Read the model definition and answer for the solid it produces. Units are mm, in the model's axes. A direction names the side the tool comes from. Round coordinates to 2 decimals unless told otherwise and drop trailing zeros. Loops run counter-clockwise (first coordinate to the right, second up) from the corner with the lowest first, then second, coordinate; pieces in that order, holes last. Notation, with made-up numbers: (-22, -4.75) - (-6, -4.75) arc R18 cw to (-6, 20.25) - close; hole circle Ø2 at (-22.75, 58). An arc over 180 degrees is marked (long way). Use one line per item in the form item = value. Start each with the question number.
```python
from build123d import *

# Parameters (mm, degrees)
SKETCH1_R           = 2.5
BOSS_EXTRUDE1_DEPTH = 300
SKETCH2_W           = 20
SKETCH2_H           = 180
CUT_EXTRUDE1_DEPTH  = 30


with BuildPart() as part:
    # Sketch1 → Boss-Extrude1 (new body)
    with BuildSketch(Plane(origin=(0, 0, 0), x_dir=(-1, 0, 0), z_dir=(0, 0, -1))):
        with BuildLine():
            Line((-20, 19), (-20, 13.2))
            Line((-20, 13.2), (-18.2, 13.2))
            Line((-18.2, 13.2), (-18.2, 14.95))
            ThreePointArc((-18.2, 14.95), (-18.053553391, 15.303553391), (-17.7, 15.45))
            Line((-17.7, 15.45), (-16.607106781, 15.45))
            ThreePointArc((-16.607106781, 15.45), (-16.415765065, 15.411939766), (-16.253553391, 15.303553391))
            Line((-16.253553391, 15.303553391), (-14.046446609, 13.096446609))
            ThreePointArc((-14.046446609, 13.096446609), (-13.938060234, 12.934234935), (-13.9, 12.742893219))
            Line((-13.9, 12.742893219), (-13.9, 7.257106781))
            ThreePointArc((-13.9, 7.257106781), (-13.938060234, 7.065765065), (-14.046446609, 6.903553391))
            Line((-14.046446609, 6.903553391), (-16.253553391, 4.696446609))
            ThreePointArc((-16.253553391, 4.696446609), (-16.415765065, 4.588060234), (-16.607106781, 4.55))
            Line((-16.607106781, 4.55), (-17.7, 4.55))
            ThreePointArc((-17.7, 4.55), (-18.053553391, 4.696446609), (-18.2, 5.05))
            Line((-18.2, 5.05), (-18.2, 6.8))
            Line((-18.2, 6.8), (-20, 6.8))
            Line((-20, 6.8), (-20, 1))
            ThreePointArc((-20, 1), (-19.707106781, 0.292893219), (-19, 0))
            Line((-19, 0), (-13.2, 0))
            Line((-13.2, 0), (-13.2, 1.8))
            Line((-13.2, 1.8), (-14.95, 1.8))
            ThreePointArc((-14.95, 1.8), (-15.303553391, 1.946446609), (-15.45, 2.3))
            Line((-15.45, 2.3), (-15.45, 3.392893219))
            ThreePointArc((-15.45, 3.392893219), (-15.411939766, 3.584234935), (-15.303553391, 3.746446609))
            Line((-15.303553391, 3.746446609), (-13.096446609, 5.953553391))
            ThreePointArc((-13.096446609, 5.953553391), (-12.934234935, 6.061939766), (-12.742893219, 6.1))
            Line((-12.742893219, 6.1), (-7.257106781, 6.1))
            ThreePointArc((-7.257106781, 6.1), (-7.065765065, 6.061939766), (-6.903553391, 5.953553391))
            Line((-6.903553391, 5.953553391), (-4.696446609, 3.746446609))
            ThreePointArc((-4.696446609, 3.746446609), (-4.588060234, 3.584234935), (-4.55, 3.392893219))
            Line((-4.55, 3.392893219), (-4.55, 2.3))
            ThreePointArc((-4.55, 2.3), (-4.696446609, 1.946446609), (-5.05, 1.8))
            Line((-5.05, 1.8), (-6.8, 1.8))
            Line((-6.8, 1.8), (-6.8, 0))
            Line((-6.8, 0), (-1, 0))
            ThreePointArc((-1, 0), (-0.292893219, 0.292893219), (0, 1))
            Line((0, 1), (0, 6.8))
            Line((0, 6.8), (-1.8, 6.8))
            Line((-1.8, 6.8), (-1.8, 5.05))
            ThreePointArc((-1.8, 5.05), (-1.946446609, 4.696446609), (-2.3, 4.55))
            Line((-2.3, 4.55), (-3.392893219, 4.55))
            ThreePointArc((-3.392893219, 4.55), (-3.584234935, 4.588060234), (-3.746446609, 4.696446609))
            Line((-3.746446609, 4.696446609), (-5.953553391, 6.903553391))
            ThreePointArc((-5.953553391, 6.903553391), (-6.061939766, 7.065765065), (-6.1, 7.257106781))
            Line((-6.1, 7.257106781), (-6.1, 12.742893219))
            ThreePointArc((-6.1, 12.742893219), (-6.061939766, 12.934234935), (-5.953553391, 13.096446609))
            Line((-5.953553391, 13.096446609), (-3.746446609, 15.303553391))
            ThreePointArc((-3.746446609, 15.303553391), (-3.584234935, 15.411939766), (-3.392893219, 15.45))
            Line((-3.392893219, 15.45), (-2.3, 15.45))
            ThreePointArc((-2.3, 15.45), (-1.946446609, 15.303553391), (-1.8, 14.95))
            Line((-1.8, 14.95), (-1.8, 13.2))
            Line((-1.8, 13.2), (0, 13.2))
            Line((0, 13.2), (0, 19))
            ThreePointArc((0, 19), (-0.292893219, 19.707106781), (-1, 20))
            Line((-1, 20), (-6.8, 20))
            Line((-6.8, 20), (-6.8, 18.2))
            Line((-6.8, 18.2), (-5.05, 18.2))
            ThreePointArc((-5.05, 18.2), (-4.696446609, 18.053553391), (-4.55, 17.7))
            Line((-4.55, 17.7), (-4.55, 16.607106781))
            ThreePointArc((-4.55, 16.607106781), (-4.588060234, 16.415765065), (-4.696446609, 16.253553391))
            Line((-4.696446609, 16.253553391), (-6.903553391, 14.046446609))
            ThreePointArc((-6.903553391, 14.046446609), (-7.065765065, 13.938060234), (-7.257106781, 13.9))
            Line((-7.257106781, 13.9), (-12.742893219, 13.9))
            ThreePointArc((-12.742893219, 13.9), (-12.934234935, 13.938060234), (-13.096446609, 14.046446609))
            Line((-13.096446609, 14.046446609), (-15.303553391, 16.253553391))
            ThreePointArc((-15.303553391, 16.253553391), (-15.411939766, 16.415765065), (-15.45, 16.607106781))
            Line((-15.45, 16.607106781), (-15.45, 17.7))
            ThreePointArc((-15.45, 17.7), (-15.303553391, 18.053553391), (-14.95, 18.2))
            Line((-14.95, 18.2), (-13.2, 18.2))
            Line((-13.2, 18.2), (-13.2, 20))
            Line((-13.2, 20), (-19, 20))
            ThreePointArc((-19, 20), (-19.707106781, 19.707106781), (-20, 19))
        make_face()
        with Locations((-10, 10)):
            Circle(SKETCH1_R, mode=Mode.SUBTRACT)
    extrude(amount=-BOSS_EXTRUDE1_DEPTH)

    # Sketch2 → Cut-Extrude1 (cut)
    with BuildSketch(Plane(origin=(0, 20, 0), x_dir=(1, 0, 0), z_dir=(0, 1, 0))):
        with Locations((10, -90)):
            Rectangle(SKETCH2_W, SKETCH2_H)
    extrude(amount=-CUT_EXTRUDE1_DEPTH, mode=Mode.SUBTRACT)


solid = part.part
```
1) A cutting plane is placed at A-A on y = 8.5. Write down the section's boundary in (x, z).
2) A cutting plane is placed at B-B on x = 10. Write down the section's boundary in (y, z), plus the area to 3 significant figures.
3) For faces 5 (the flat face through (14.22, 4.83, 239.16)), 6 (the flat face through (6.1, 10, 239)), 7 (the flat face through (10, 13.9, 239)), 8 (the flat face through (10, 6.1, 239)), determine the directions among +Z, -Z, +X, -X, +Y, -Y from which every point of the face is accessible in a straight line to the end or side of a thin tool.
4) Flat-ended cylindrical pins translate along their axes: pin 1 (3 mm diameter, centred on y = 9.5, z = 277.5, fed in from +X); pin 2 (0.9 mm diameter, centred on y = 3, z = 247.5, fed in from -X). Find the tip coordinate at first contact, or state that the pin passes through.
5) Straight lines are drawn through the part: line 1 (X direction, y = 2.25, z = 187); line 2 (Y direction, x = 10, z = 229); line 3 (X direction, y = 19, z = 222.5). For each, find the intervals that lie inside material, in ascending order. Write a range as from..to.
6) Determine the mould class of faces 1 (the cylindrical face through (10.54, 7.56, 239.16)), 2 (the flat face through (4, 0, 239)), 3 (the flat face through (0, 16, 239)), 4 (the flat face through (4.87, 14.18, 239.16)) for opening direction X: +X half, -X half, draft (parallel to the pull), parting line (faces both ways), or undercut.
Checks:
q1.outline = (6.1, 180) - (8, 180) - (8, 300) - (6.1, 300) - close; (12, 180) - (13.9, 180) - (13.9, 300) - (12, 300) - close
q2.outline = (6.1, 180) - (7.5, 180) - (7.5, 300) - (6.1, 300) - close; (12.5, 180) - (13.9, 180) - (13.9, 300) - (12.5, 300) - close
q2.area = 336 mm²
q3.face_5 = +Z, -Z
q3.face_6 = +Z, -Z, -X
q3.face_7 = +Z, -Z, +Y
q3.face_8 = +Z, -Z, -Y
q4.pin_1 = 13.9
q4.pin_2 = 0
q5.line_1 = 0..4.55, 15.45..20
q5.line_2 = 6.1..7.5, 12.5..13.9
q5.line_3 = 0..6.8, 13.2..20
q6.face_1 = undercut
q6.face_2 = draft
q6.face_3 = -X half
q6.face_4 = undercut
